Read the model definition and answer for the solid it produces. Units are mm, in the model's axes. A direction names the side the tool comes from. Coordinates: 2 decimals unless noted, no trailing zeros. Write each loop counter-clockwise with the first axis right and the second up, starting at its lowest first coordinate (ties: lowest second). Pieces come first, ordered by that corner, then holes.
Item 1: Each of these flat-tipped pins is pushed along its axis until it touches: P1, Ø7, axis at y = 16, z = 8.5, coming from the -X side; P2, Ø3, axis at x = 14, z = 12, coming from the +Y side; P3, Ø4, axis at x = 88, z = -15, coming from the -Y side; P4, Ø8, axis at x = 69.5, z = -1, coming from the -Y side. Where does it stop, or does it pass through?
Item 2: Section C-C (z = 20) is taken. Give the vertices of the cut face in (x, y).
Item 3: A tool of negligible diameter and unlimited length cuts with its end or side. For faces 4 (the face through (19, 80, 10)), 5 (the face through (85.27, 11.1, 13.8)), 6 (the face through (87, 81.5, 6)), from which of +Z, -Z, +X, -X, +Y, -Y can it reach the whole face along a straight path? Write none if from no direction.
Item 4: Section D-D (x = 68.5) is taken. Give the vertices of the cut face in (y, z).
Item 5: Determine the mould class of faces 1 (the face through (85.3, 14.35, -15.65)), 2 (the face through (14, 80, 5)), 3 (the face through (14, 89, 28)) for opening direction X: released by +X, released by -X, zero draft, split by the parting line, or undercut.
Item 6: Section A-A (x = 53) is taken. Give the vertices of the cut face in (y, z).
Item 7: Straight lines are drawn through the part: probe 1 along X at (y, z) = (37, 4); probe 2 along X at (y, z) = (92.5, 8.5); probe 3 along Y at (x, z) = (66, 6). For each, find the intervals that lie inside material, in ascending order.
Item 8: Section B-B (y = 84) is taken. Give the vertices of the cut face in (x, z), then the cut area to 3 significant figures.
from build123d import *

# Parameters (mm, degrees)
F0_W     = 102
F0_H     = 102
F0_W_2   = 9.5
F0_H_2   = 4.4
F0_W_3   = 10.1
F0_H_3   = 19
F0_W_4   = 31
F0_H_4   = 9
F0_W_5   = 28.7
F0_H_5   = 12.6
F0_W_6   = 9
F0_H_6   = 61
F0_W_7   = 42
F0_H_7   = 21.8
F1_DEPTH = 1.5
F2_DEPTH = 30.2
F3_DEPTH = 28
F4_DEPTH = 0.1
F5_DEPTH = 13
F6_DEPTH = 10
F7_DEPTH = 7.7
F8_DEPTH = 15.7


with BuildPart() as f1:
    # F0 (on Top) → F1 (new body)
    with BuildSketch(Plane.XY):
        with Locations((51, 51)):
            Rectangle(F0_W, F0_H)
        Polygon((10.1472232503, 12.7), (12.0236116251, 15.95), (15.7763883749, 15.95), (17.6527767497, 12.7), (15.7763883749, 9.45), (12.0236116251, 9.45), align=None, mode=Mode.SUBTRACT)
        with Locations((9.15, 31.2)):
            Rectangle(F0_W_2, F0_H_2, mode=Mode.SUBTRACT)
        with Locations((20.05, 50.9)):
            Rectangle(F0_W_3, F0_H_3, mode=Mode.SUBTRACT)
        with Locations((51, 15.5)):
            Rectangle(F0_W_4, F0_H_4, mode=Mode.SUBTRACT)
        Polygon((86.2236116251, 15.95), (89.9763883749, 15.95), (91.8527767497, 12.7), (89.9763883749, 9.45), (86.2236116251, 9.45), (84.3472232503, 12.7), align=None, mode=Mode.SUBTRACT)
        with Locations((63.95, 42.2)):
            Rectangle(F0_W_5, F0_H_5, mode=Mode.SUBTRACT)
        with Locations((18.75, 79.8)):
            Rectangle(F0_W_2, F0_H_2, mode=Mode.SUBTRACT)
        Polygon((15.7763883749, 92.55), (17.6527767497, 89.3), (15.7763883749, 86.05), (12.0236116251, 86.05), (10.1472232503, 89.3), (12.0236116251, 92.55), align=None, mode=Mode.SUBTRACT)
        with Locations((87.5, 51)):
            Rectangle(F0_W_6, F0_H_6, mode=Mode.SUBTRACT)
        with Locations((51, 87.1)):
            Rectangle(F0_W_7, F0_H_7, mode=Mode.SUBTRACT)
        Polygon((89.9763883749, 92.55), (91.8527767497, 89.3), (89.9763883749, 86.05), (86.2236116251, 86.05), (84.3472232503, 89.3), (86.2236116251, 92.55), align=None, mode=Mode.SUBTRACT)
        with Locations((51, 87.1)):
            Rectangle(F0_W_7, F0_H_7)
        with Locations((87.5, 51)):
            Rectangle(F0_W_6, F0_H_6)
        with Locations((63.95, 42.2)):
            Rectangle(F0_W_5, F0_H_5)
        with Locations((51, 15.5)):
            Rectangle(F0_W_4, F0_H_4)
        with Locations((20.05, 50.9)):
            Rectangle(F0_W_3, F0_H_3)
        with Locations((9.15, 31.2)):
            Rectangle(F0_W_2, F0_H_2)
        with Locations((18.75, 79.8)):
            Rectangle(F0_W_2, F0_H_2)
        Polygon((91.8527767497, 12.7), (89.9763883749, 15.95), (86.2236116251, 15.95), (84.3472232503, 12.7), (86.2236116251, 9.45), (89.9763883749, 9.45), align=None)
        Polygon((15.7763883749, 15.95), (12.0236116251, 15.95), (10.1472232503, 12.7), (12.0236116251, 9.45), (15.7763883749, 9.45), (17.6527767497, 12.7), align=None)
        Polygon((15.7763883749, 86.05), (17.6527767497, 89.3), (15.7763883749, 92.55), (12.0236116251, 92.55), (10.1472232503, 89.3), (12.0236116251, 86.05), align=None)
        Polygon((89.9763883749, 86.05), (91.8527767497, 89.3), (89.9763883749, 92.55), (86.2236116251, 92.55), (84.3472232503, 89.3), (86.2236116251, 86.05), align=None)
    extrude(amount=-F1_DEPTH)

    # F0 (on Top) → F2 (join)
    with BuildSketch(Plane.XY):
        Polygon((15.7763883749, 15.95), (12.0236116251, 15.95), (10.1472232503, 12.7), (12.0236116251, 9.45), (15.7763883749, 9.45), (17.6527767497, 12.7), align=None)
        Polygon((15.7763883749, 86.05), (17.6527767497, 89.3), (15.7763883749, 92.55), (12.0236116251, 92.55), (10.1472232503, 89.3), (12.0236116251, 86.05), align=None)
        Polygon((89.9763883749, 86.05), (91.8527767497, 89.3), (89.9763883749, 92.55), (86.2236116251, 92.55), (84.3472232503, 89.3), (86.2236116251, 86.05), align=None)
        Polygon((91.8527767497, 12.7), (89.9763883749, 15.95), (86.2236116251, 15.95), (84.3472232503, 12.7), (86.2236116251, 9.45), (89.9763883749, 9.45), align=None)
    extrude(amount=-F2_DEPTH)

    # F0 (on Top) → F3 (join)
    with BuildSketch(Plane.XY):
        Polygon((15.7763883749, 86.05), (17.6527767497, 89.3), (15.7763883749, 92.55), (12.0236116251, 92.55), (10.1472232503, 89.3), (12.0236116251, 86.05), align=None)
        Polygon((89.9763883749, 86.05), (91.8527767497, 89.3), (89.9763883749, 92.55), (86.2236116251, 92.55), (84.3472232503, 89.3), (86.2236116251, 86.05), align=None)
        Polygon((91.8527767497, 12.7), (89.9763883749, 15.95), (86.2236116251, 15.95), (84.3472232503, 12.7), (86.2236116251, 9.45), (89.9763883749, 9.45), align=None)
        Polygon((15.7763883749, 15.95), (12.0236116251, 15.95), (10.1472232503, 12.7), (12.0236116251, 9.45), (15.7763883749, 9.45), (17.6527767497, 12.7), align=None)
    extrude(amount=F3_DEPTH)

    # F0 (on Top) → F4 (join)
    with BuildSketch(Plane.XY):
        with Locations((51, 87.1)):
            Rectangle(F0_W_7, F0_H_7)
    extrude(amount=F4_DEPTH)

    # F0 (on Top) → F5 (join)
    with BuildSketch(Plane.XY):
        with Locations((51, 15.5)):
            Rectangle(F0_W_4, F0_H_4)
        with Locations((87.5, 51)):
            Rectangle(F0_W_6, F0_H_6)
    extrude(amount=F5_DEPTH)

    # F0 (on Top) → F6 (join)
    with BuildSketch(Plane.XY):
        with Locations((9.15, 31.2)):
            Rectangle(F0_W_2, F0_H_2)
        with Locations((18.75, 79.8)):
            Rectangle(F0_W_2, F0_H_2)
    extrude(amount=F6_DEPTH)

    # F0 (on Top) → F7 (join)
    with BuildSketch(Plane.XY):
        with Locations((20.05, 50.9)):
            Rectangle(F0_W_3, F0_H_3)
    extrude(amount=F7_DEPTH)

    # F0 (on Top) → F8 (join)
    with BuildSketch(Plane.XY):
        with Locations((63.95, 42.2)):
            Rectangle(F0_W_5, F0_H_5)
    extrude(amount=F8_DEPTH)


solid = f1.part
Established:
1. P1: stops at x = 10.15
1. P2: stops at y = 92.55
1. P3: stops at y = 9.45
1. P4: stops at y = 0
2. outline: (10.15, 12.7) - (12.02, 9.45) - (15.78, 9.45) - (17.65, 12.7) - (15.78, 15.95) - (12.02, 15.95) - close; (10.15, 89.3) - (12.02, 86.05) - (15.78, 86.05) - (17.65, 89.3) - (15.78, 92.55) - (12.02, 92.55) - close; (84.35, 12.7) - (86.22, 9.45) - (89.98, 9.45) - (91.85, 12.7) - (89.98, 15.95) - (86.22, 15.95) - close; (84.35, 89.3) - (86.22, 86.05) - (89.98, 86.05) - (91.85, 89.3) - (89.98, 92.55) - (86.22, 92.55) - close
3. face 4: +Z, -X
3. face 5: +Z, -Y
3. face 6: +Z, +X
4. outline: (0, -1.5) - (102, -1.5) - (102, 0) - (98, 0) - (98, 0.1) - (76.2, 0.1) - (76.2, 0) - (48.5, 0) - (48.5, 15.7) - (35.9, 15.7) - (35.9, 0) - (0, 0) - close
5. face 1: undercut
5. face 2: released by -X
5. face 3: zero draft
6. outline: (0, -1.5) - (102, -1.5) - (102, 0) - (98, 0) - (98, 0.1) - (76.2, 0.1) - (76.2, 0) - (48.5, 0) - (48.5, 15.7) - (35.9, 15.7) - (35.9, 0) - (20, 0) - (20, 13) - (11, 13) - (11, 0) - (0, 0) - close
7. probe 1: x = 49.6 to 78.3, 83 to 92
7. probe 2: x = 11.99 to 15.81, 86.19 to 90.01
7. probe 3: y = 11 to 20, 35.9 to 48.5
8. outline: (0, -1.5) - (102, -1.5) - (102, 0) - (72, 0) - (72, 0.1) - (30, 0.1) - (30, 0) - (0, 0) - close
8. area: 157 mm2
